Job drawing, mm, ordinate dimensions from the low corner. One solid piece. Give positions to 0.01 mm unless a question says otherwise; leave off trailing zeros. Loops run counter-clockwise (first coordinate to the right, second up) from the corner with the lowest first, then second, coordinate; pieces in that order, holes last. Notation, with made-up numbers: (-21, -14.5) - (12, -14.5) arc R35 cw to (12, 21.5) - close; hole circle Ø3 at (-14, -4.75). An arc over 180 degrees is marked (long way). Use a Markdown table: item, result.
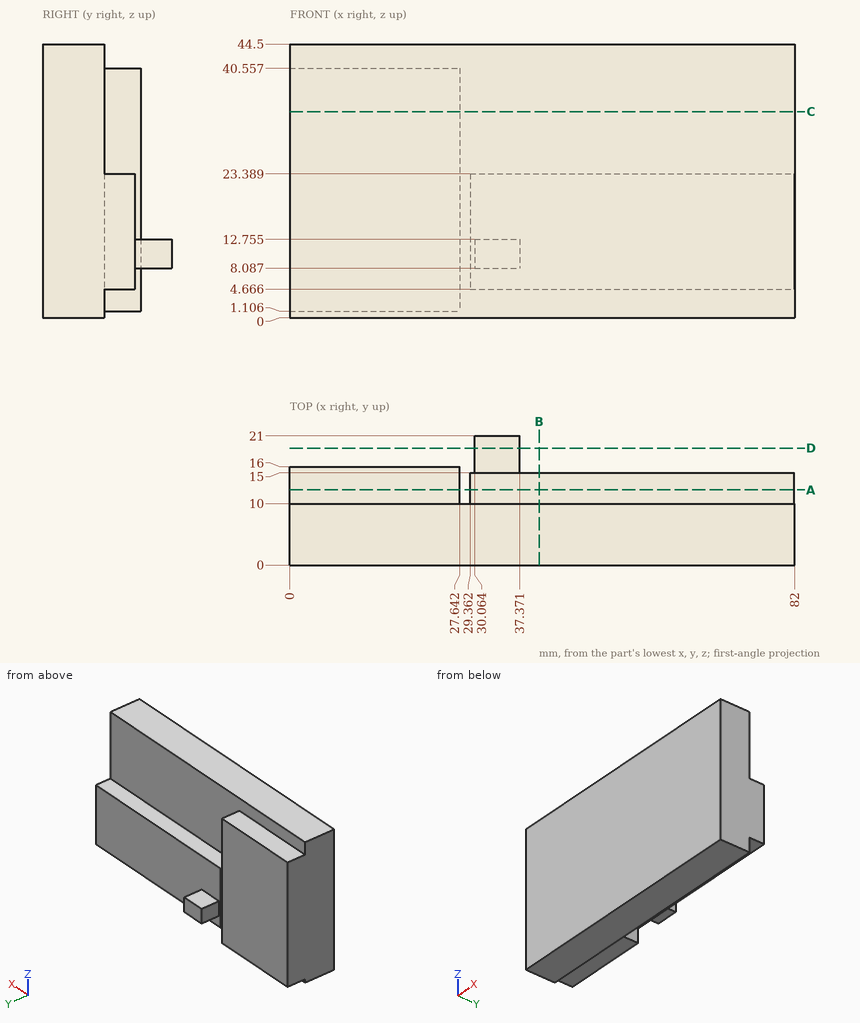
(1) Pin check, flat tips, straight feed: P1, Ø1.4, axis at y = 17.5, z = 9.5, coming from the +X side; P2, Ø2, axis at x = 72, z = 32, coming from the +Y side; P3, Ø20.5, axis at x = 60, z = 15.5, coming from the +Y side; P4, Ø5, axis at x = 53.5, y = 18.5, coming from the -Z side. Stop position of each tip, or through.
Computed:
| item | result |
|---|---|
| P1 | x = 37.37 |
| P2 | y = 10 |
| P3 | y = 15 |
| P4 | through |
(2) Slice it at D-D, the plane y = 19. Write the cut outline in (x, z) (1 decimal).
Computed:
| item | result |
|---|---|
| outline | (30.1, 8.1) - (37.4, 8.1) - (37.4, 12.8) - (30.1, 12.8) - close |
(3) Slice it at B-B, the plane x = 40.5. Write the cut outline in (y, z).
Computed:
| item | result |
|---|---|
| outline | (0, 0) - (10, 0) - (10, 4.67) - (15, 4.67) - (15, 23.39) - (10, 23.39) - (10, 44.5) - (0, 44.5) - close |
(4) Drill centre lines: probe 1 along Z at (x, y) = (40.5, 11.25); probe 2 along X at (y, z) = (17.5, 9); probe 3 along Y at (x, z) = (32, 14). Where is each one in solid material? Low to high. Write a range as [from, to].
Computed:
| item | result |
|---|---|
| probe 1 | [4.67, 23.39] |
| probe 2 | [30.06, 37.37] |
| probe 3 | [0, 15] |
(5) Slice it at C-C, the plane z = 33.5. Write the cut outline in (x, y), plus the area to 3 significant figures.
Computed:
| item | result |
|---|---|
| outline | (0, 0) - (82, 0) - (82, 10) - (27.64, 10) - (27.64, 16) - (0, 16) - close |
| area | 986 mm² |
(6) Slice it at A-A, the plane y = 12.25. Write the cut outline in (x, z).
Computed:
| item | result |
|---|---|
| outline | (0, 1.11) - (27.64, 1.11) - (27.64, 40.56) - (0, 40.56) - close; (29.36, 4.67) - (82, 4.67) - (82, 23.39) - (29.36, 23.39) - close |
